```python
from build123d import *

# Parameters (mm, degrees)
SKETCH1_W           = 80
SKETCH1_H           = 95
BOSS_EXTRUDE1_DEPTH = 10
SKETCH2_W           = 10
SKETCH2_H           = 10
CUT_EXTRUDE1_DEPTH  = 10
SKETCH3_W           = 80
SKETCH3_H           = 5
BOSS_EXTRUDE2_DEPTH = 5
CUT_EXTRUDE2_DEPTH  = 1.5
SKETCH5_W           = 39
SKETCH5_H           = 17
CUT_EXTRUDE3_DEPTH  = 8.5
SKETCH6_W           = 9.5
SKETCH6_H           = 5
BOSS_EXTRUDE3_DEPTH = 100
SKETCH7_W           = 73
SKETCH7_H           = 8
BOSS_EXTRUDE4_DEPTH = 5
SKETCH8_W           = 80
SKETCH8_H           = 1
CUT_EXTRUDE4_DEPTH  = 5
CUT_EXTRUDE5_DEPTH  = 10


with BuildPart() as part:
    # Sketch1 → Boss-Extrude1 (new body)
    with BuildSketch(Plane(origin=(0, 0, 0), x_dir=(1, 0, 0), z_dir=(0, 1, 0))):
        Rectangle(SKETCH1_W, SKETCH1_H)
    extrude(amount=BOSS_EXTRUDE1_DEPTH)

    # Sketch2 → Cut-Extrude1 (cut)
    with BuildSketch(Plane(origin=(0, 10, 0), x_dir=(1, 0, 0), z_dir=(0, 1, 0))):
        with Locations((-35, 42.5)):
            Rectangle(SKETCH2_W, SKETCH2_H)
        with Locations((35, 42.5)):
            Rectangle(SKETCH2_W, SKETCH2_H)
    extrude(amount=-CUT_EXTRUDE1_DEPTH, mode=Mode.SUBTRACT)

    # Sketch3 → Boss-Extrude2 (add)
    with BuildSketch(Plane(origin=(0, 10, 0), x_dir=(1, 0, 0), z_dir=(0, 1, 0))):
        with Locations((0, -45)):
            Rectangle(SKETCH3_W, SKETCH3_H)
    extrude(amount=BOSS_EXTRUDE2_DEPTH)

    # Sketch4 → Cut-Extrude2 (cut)
    with BuildSketch(Plane(origin=(0, 10, 0), x_dir=(1, 0, 0), z_dir=(0, 1, 0))):
        Polygon((-21, -13), (21, -13), (21, 8), (6.491381871, 8), (6.5, 47.5), (-6.5, 47.5), (-6.5, 8), (-21, 8), align=None)
    extrude(amount=-CUT_EXTRUDE2_DEPTH, mode=Mode.SUBTRACT)

    # Sketch5 → Cut-Extrude3 (cut)
    with BuildSketch(Plane(origin=(0, 8.5, 0), x_dir=(1, 0, 0), z_dir=(0, 1, 0))):
        with Locations((0, -2.5)):
            Rectangle(SKETCH5_W, SKETCH5_H)
    extrude(amount=-CUT_EXTRUDE3_DEPTH, mode=Mode.SUBTRACT)

    # Sketch6 → Boss-Extrude3 (add)
    with BuildSketch(Plane(origin=(0, 10, 0), x_dir=(1, 0, 0), z_dir=(0, 1, 0))):
        with Locations((-24.75, 42.5)):
            Rectangle(SKETCH6_W, SKETCH6_H)
        with Locations((24.75, 42.5)):
            Rectangle(SKETCH6_W, SKETCH6_H)
    extrude(amount=BOSS_EXTRUDE3_DEPTH)

    # Sketch7 → Boss-Extrude4 (add)
    with BuildSketch(Plane.XY.offset(-40)):
        with Locations((0, 35)):
            Rectangle(SKETCH7_W, SKETCH7_H)
        with Locations((0, 75)):
            Rectangle(SKETCH7_W, SKETCH7_H)
    extrude(amount=-BOSS_EXTRUDE4_DEPTH)

    # Sketch8 → Cut-Extrude4 (cut)
    with BuildSketch(Plane(origin=(0, 15, 0), x_dir=(1, 0, 0), z_dir=(0, 1, 0))):
        with Locations((0, -43)):
            Rectangle(SKETCH8_W, SKETCH8_H)
    extrude(amount=-CUT_EXTRUDE4_DEPTH, mode=Mode.SUBTRACT)

    # Sketch9 → Cut-Extrude5 (cut)
    with BuildSketch(Plane(origin=(0, 10, 0), x_dir=(1, 0, 0), z_dir=(0, 1, 0))):
        Polygon((30, 47.5), (29.5, 47.5), (29.5, 37), (40, 37), (40, 37.5), (30, 37.5), align=None)
        Polygon((-40, 37.5), (-30, 37.5), (-30, 47.5), (-29.5, 47.5), (-29.5, 37), (-40, 37), align=None)
    extrude(amount=-CUT_EXTRUDE5_DEPTH, mode=Mode.SUBTRACT)


solid = part.part
```
For this review, take the finished solid that the model builds, in its own axes (mm). A direction names the side the tool comes from. Round coordinates to 2 decimals unless told otherwise and drop trailing zeros. Order: outer loops, then holes, each group sorted by start corner. A loop starts at its lowest first (then second) coordinate and runs counter-clockwise, first axis right, second up.
Q1. We need section A-A, the plane x = 9. Give the boundary of the cut face in (y, z), plus the area to 3 significant figures.
Findings below:
outline: (0, -47.5) - (10, -47.5) - (10, -8) - (8.5, -8) - (8.5, -6) - (0, -6) - close; (0, 11) - (8.5, 11) - (8.5, 13) - (10, 13) - (10, 43.5) - (15, 43.5) - (15, 47.5) - (0, 47.5) - close; (31, -45) - (39, -45) - (39, -40) - (31, -40) - close; (71, -45) - (79, -45) - (79, -40) - (71, -40) - close
area: 874 mm2
Q2. We need section B-B, the plane y = 84. Give the boundary of the cut face in (x, z).
Findings below:
outline: (-29.5, -45) - (-20, -45) - (-20, -40) - (-29.5, -40) - close; (20, -45) - (29.5, -45) - (29.5, -40) - (20, -40) - close
Q3. Insertion check: P1, Ø5.5, axis at y = 76.5, z = -43, coming from the -X side; P2, Ø2.5, axis at y = 22.5, z = -43, coming from the +X side; P3, Ø4, axis at x = -26, y = 59.5, coming from the +Z side. Each pin has a flat end and moves straight along its axis. Give the tip position at first contact, or say it passes through.
Findings below:
P1: stops at x = -36.5
P2: stops at x = 29.5
P3: stops at z = -40
Q4. Machinability: for faces 5 (the flat face through (33, 79, -42)), 6 (the flat face through (-33, 79, -42)), 7 (the flat face through (-20, 94, -42)), 8 (the flat face through (29.5, 55, -42)), which of the approach directions +Z, -Z, +X, -X, +Y, -Y give a long, thin tool a straight path to every point of the face, cutting with its end or side? Answer none if there is none.
Findings below:
face 5: +Z, -Z, +X, +Y
face 6: +Z, -Z, -X, +Y
face 7: +Z, -Z, +Y
face 8: +Z, -Z, +X
Q5. Wall thickness on line 1 (Y direction, x = -32, z = 40); line 2 (X direction, y = 6, z = 2.5); line 3 (Z direction, x = -24, y = 35): over which ranges is each line inside the solid? List them lowest first.
Findings below:
line 1: y = 0 to 10
line 2: x = -40 to -19.5, 19.5 to 40
line 3: z = -45 to -40
Q6. We need section D-D, the plane z = -19. Give the boundary of the cut face in (x, y), plus the area to 3 significant figures.
Findings below:
outline: (-40, 0) - (40, 0) - (40, 10) - (6.49, 10) - (6.49, 8.5) - (-6.5, 8.5) - (-6.5, 10) - (-40, 10) - close
area: 781 mm2
Q7. Mouldability with a two-part tool opening along X and no side actions: class faces 1 (the flat face through (29.5, 12, -42)), 2 (the flat face through (-29.5, 12, -42)), 3 (the flat face through (-1, 72, -45)), 4 (the flat face through (20, 20, -42)) as pulls with the +X half, pulls with the -X half, needs draft (parallel to the pull), parting line crosses it, or undercut.
Findings below:
face 1: pulls with the +X half
face 2: pulls with the -X half
face 3: needs draft
face 4: undercut
Q8. We need section C-C, the plane x = 24. Give the boundary of the cut face in (y, z).
Findings below:
outline: (0, -47.5) - (10, -47.5) - (10, -45) - (110, -45) - (110, -40) - (10, -40) - (10, 43.5) - (15, 43.5) - (15, 47.5) - (0, 47.5) - close
